from build123d import *

# Parameters (mm, degrees)
SKETCH1_R           = 50
BOSS_EXTRUDE1_DEPTH = 28
SKETCH4_R           = 53.870598216
SKETCH4_R_2         = 45
CUT_EXTRUDE1_DEPTH  = 20
SKETCH5_R           = 37.1
CUT_EXTRUDE2_DEPTH  = 46.383141605
SKETCH6_R           = 43
SKETCH6_R_2         = 39.1
CUT_EXTRUDE3_DEPTH  = 2
SKETCH7_R           = 1.4
CUT_EXTRUDE4_DEPTH  = 7
EXTRUDE_THIN1_START = 8
SKETCH8_R           = 50
SKETCH8_R_2         = 48.4
EXTRUDE_THIN1_DEPTH = 8
SKETCH9_R           = 48.4
SKETCH9_R_2         = 44.1
SKETCH9_R_3         = 1.4
CUT_EXTRUDE5_DEPTH  = 2
SKETCH10_W          = 2.3
SKETCH10_H          = 3.9
SKETCH11_R          = 1.356303205
CUT_EXTRUDE7_DEPTH  = 5


with BuildPart() as part:
    # Sketch1 → Boss-Extrude1 (new body)
    with BuildSketch(Plane.XY):
        Circle(SKETCH1_R)
    extrude(amount=-BOSS_EXTRUDE1_DEPTH)

    # Sketch4 → Cut-Extrude1 (cut)
    with BuildSketch(Plane(origin=(0, 0, -28), x_dir=(-1, 0, 0), z_dir=(0, 0, -1))):
        Circle(SKETCH4_R)
        Circle(SKETCH4_R_2, mode=Mode.SUBTRACT)
    extrude(amount=-CUT_EXTRUDE1_DEPTH, mode=Mode.SUBTRACT)

    # Sketch5 → Cut-Extrude2 (cut)
    with BuildSketch(Plane(origin=(0, 0, -28), x_dir=(-1, 0, 0), z_dir=(0, 0, -1))):
        Circle(SKETCH5_R)
    extrude(amount=-CUT_EXTRUDE2_DEPTH, mode=Mode.SUBTRACT)

    # Sketch6 → Cut-Extrude3 (cut)
    with BuildSketch(Plane.XY):
        Circle(SKETCH6_R)
        Circle(SKETCH6_R_2, mode=Mode.SUBTRACT)
    extrude(amount=-CUT_EXTRUDE3_DEPTH, mode=Mode.SUBTRACT)

    # Sketch7 → Cut-Extrude4 (cut)
    with BuildSketch(Plane.XY):
        with Locations((0, 46)):
            Circle(SKETCH7_R)
        with Locations((39.837168574, 23)):
            Circle(SKETCH7_R)
        with Locations((39.837168574, -23)):
            Circle(SKETCH7_R)
        with Locations((0, -46)):
            Circle(SKETCH7_R)
        with Locations((-39.837168574, -23)):
            Circle(SKETCH7_R)
        with Locations((-39.837168574, 23)):
            Circle(SKETCH7_R)
    extrude(amount=-CUT_EXTRUDE4_DEPTH, mode=Mode.SUBTRACT)

    # Sketch8 → Extrude-Thin1 (add)
    with BuildSketch(Plane.XY.offset(EXTRUDE_THIN1_START)):
        Circle(SKETCH8_R)
        Circle(SKETCH8_R_2, mode=Mode.SUBTRACT)
    extrude(amount=-EXTRUDE_THIN1_DEPTH)

    # Sketch9 → Cut-Extrude5 (cut)
    with BuildSketch(Plane.XY):
        Circle(SKETCH9_R)
        Circle(SKETCH9_R_2, mode=Mode.SUBTRACT)
        with Locations((-39.837168574, -23)):
            Circle(SKETCH9_R_3, mode=Mode.SUBTRACT)
        with Locations((-39.837168574, 23)):
            Circle(SKETCH9_R_3, mode=Mode.SUBTRACT)
        with Locations((0, -46)):
            Circle(SKETCH9_R_3, mode=Mode.SUBTRACT)
        with Locations((0, 46)):
            Circle(SKETCH9_R_3, mode=Mode.SUBTRACT)
        with Locations((39.837168574, -23)):
            Circle(SKETCH9_R_3, mode=Mode.SUBTRACT)
        with Locations((39.837168574, 23)):
            Circle(SKETCH9_R_3, mode=Mode.SUBTRACT)
    extrude(amount=-CUT_EXTRUDE5_DEPTH, mode=Mode.SUBTRACT)

    # Sketch10 → Cut-Revolve1 (revolve, cut)
    with BuildSketch(Plane(origin=(0, 0, 0), x_dir=(1, 0, 0), z_dir=(0, 1, 0)), mode=Mode.PRIVATE) as cut_revolve1_sk:
        with Locations((-43.85, 11.95)):
            Rectangle(SKETCH10_W, SKETCH10_H)
        with Locations((-43.85, 19.201350281)):
            Rectangle(SKETCH10_W, SKETCH10_H)
    revolve(cut_revolve1_sk.sketch.rotate(Axis((0, 0, 0), (0, 0, -1)), 180), axis=Axis((0, 0, 0), (0, 0, -1)), mode=Mode.SUBTRACT)

    # Sketch11 → Cut-Extrude7 (cut)
    with BuildSketch(Plane(origin=(0, 0, -28), x_dir=(-1, 0, 0), z_dir=(0, 0, -1))):
        with Locations((0, 40.874722667)):
            Circle(SKETCH11_R)
        with Locations((40.874722667, 0)):
            Circle(SKETCH11_R)
        with Locations((0, -40.874722667)):
            Circle(SKETCH11_R)
        with Locations((-40.874722667, 0)):
            Circle(SKETCH11_R)
    extrude(amount=-CUT_EXTRUDE7_DEPTH, mode=Mode.SUBTRACT)


solid = part.part
Build history of the part. All positions in model axes, mm. A direction names the side the tool comes from. Give positions to 0.01 mm unless a question says otherwise; leave off trailing zeros. Put each result on its own line as item: value.
Item 1: Drop flat-ended pins along their axis: pin 1 Ø1.4 at (x, y) = (-40, -22.5) entering from +Z; pin 2 Ø3 at (x, y) = (41, 0) entering from -Z; pin 3 Ø3 at (x, z) = (-39, -3) entering from -Y; pin 4 Ø3 at (x, y) = (0, -46.5) entering from +Z. Give the stop position or say it passes through.
Results are:
pin 1: z = -7
pin 2: z = -28
pin 3: y = -33.07
pin 4: z = -2
Item 2: Pull direction Y, two halves, no side cores. Call faces 1 (the face through (16, 40, -10)), 2 (the face through (19.703, 37.882, -19.229)), 3 (the face through (41.13, -23.54, -4.46)): +Y half, -Y half, draft (parallel to the pull), parting line (faces both ways), or undercut.
Results are:
face 1: draft
face 2: parting line
face 3: undercut
Item 3: Which spindle directions (+Z, -Z, +X, -X, +Y, -Y) get a long thin tool onto all of the face, cutting with end or side? Do faces 4 (the face through (-20.765, -39.923, -9.014)), 5 (the face through (19.703, 37.882, -11.977)), 6 (the face through (10, -42, 0)), 7 (the face through (4.83, 36.784, -14.196)). Say none if no direction does.
Results are:
face 4: -Z
face 5: none
face 6: +Z
face 7: +Z, -Z
Item 4: Wall check: probe 1 along Y at (x, z) = (0, -5.2); probe 2 along Y at (x, z) = (0, -26.6); probe 3 along Z at (x, y) = (-30.5, -30.5). Give the ranges that are in metal, low to high.
Results are:
probe 1: -50 to -47.4, -44.6 to -37.1, 37.1 to 44.6, 47.4 to 50
probe 2: -45 to -42.23, -39.52 to -37.1, 37.1 to 39.52, 42.23 to 45
probe 3: -28 to -21.15, -17.25 to -13.9, -10 to 0
